```python
from build123d import *

# Parameters (mm, degrees)
SKETCH1_W           = 610
SKETCH1_H           = 200
SKETCH1_W_2         = 4
SKETCH1_H_2         = 20
SKETCH1_W_3         = 20
SKETCH1_H_3         = 4
BOSS_EXTRUDE1_DEPTH = 4
CUT_EXTRUDE1_DEPTH  = 10


with BuildPart() as part:
    # Sketch1 → Boss-Extrude1 (new body)
    with BuildSketch(Plane(origin=(0, 0, 0), x_dir=(1, 0, 0), z_dir=(0, 1, 0))):
        Rectangle(SKETCH1_W, SKETCH1_H)
        with Locations((-299, -85)):
            Rectangle(SKETCH1_W_2, SKETCH1_H_2, mode=Mode.SUBTRACT)
        with Locations((-299, 85)):
            Rectangle(SKETCH1_W_2, SKETCH1_H_2, mode=Mode.SUBTRACT)
        with Locations((-299, 0)):
            Rectangle(SKETCH1_W_2, SKETCH1_H_2, mode=Mode.SUBTRACT)
        with Locations((-275, 93)):
            Rectangle(SKETCH1_W_3, SKETCH1_H_3, mode=Mode.SUBTRACT)
        with Locations((-138, 93)):
            Rectangle(SKETCH1_W_3, SKETCH1_H_3, mode=Mode.SUBTRACT)
        with Locations((-1, 93)):
            Rectangle(SKETCH1_W_3, SKETCH1_H_3, mode=Mode.SUBTRACT)
        with Locations((-1, -93)):
            Rectangle(SKETCH1_W_3, SKETCH1_H_3, mode=Mode.SUBTRACT)
        with Locations((-138, -93)):
            Rectangle(SKETCH1_W_3, SKETCH1_H_3, mode=Mode.SUBTRACT)
        with Locations((-275, -93)):
            Rectangle(SKETCH1_W_3, SKETCH1_H_3, mode=Mode.SUBTRACT)
        with Locations((-49.859697176, -81)):
            Rectangle(SKETCH1_W_2, SKETCH1_H_2, mode=Mode.SUBTRACT)
        with Locations((-49.859697176, -32)):
            Rectangle(SKETCH1_W_2, SKETCH1_H_2, mode=Mode.SUBTRACT)
        with Locations((-64.859697176, -14)):
            Rectangle(SKETCH1_W_3, SKETCH1_H_3, mode=Mode.SUBTRACT)
        with Locations((-64.859697176, 14)):
            Rectangle(SKETCH1_W_3, SKETCH1_H_3, mode=Mode.SUBTRACT)
        with Locations((-49.859697176, 32)):
            Rectangle(SKETCH1_W_2, SKETCH1_H_2, mode=Mode.SUBTRACT)
        with Locations((0, -14)):
            Rectangle(SKETCH1_W_3, SKETCH1_H_3, mode=Mode.SUBTRACT)
        with Locations((0.140302824, 14)):
            Rectangle(SKETCH1_W_3, SKETCH1_H_3, mode=Mode.SUBTRACT)
        with Locations((136, 93)):
            Rectangle(SKETCH1_W_3, SKETCH1_H_3, mode=Mode.SUBTRACT)
        with Locations((273, 93)):
            Rectangle(SKETCH1_W_3, SKETCH1_H_3, mode=Mode.SUBTRACT)
        with Locations((49.859697176, -81)):
            Rectangle(SKETCH1_W_2, SKETCH1_H_2, mode=Mode.SUBTRACT)
        with Locations((49.859697176, -32)):
            Rectangle(SKETCH1_W_2, SKETCH1_H_2, mode=Mode.SUBTRACT)
        with Locations((64.859697176, -14)):
            Rectangle(SKETCH1_W_3, SKETCH1_H_3, mode=Mode.SUBTRACT)
        with Locations((64.859697176, 14)):
            Rectangle(SKETCH1_W_3, SKETCH1_H_3, mode=Mode.SUBTRACT)
        with Locations((49.859697176, 32)):
            Rectangle(SKETCH1_W_2, SKETCH1_H_2, mode=Mode.SUBTRACT)
        with Locations((273, -93)):
            Rectangle(SKETCH1_W_3, SKETCH1_H_3, mode=Mode.SUBTRACT)
        with Locations((136, -93)):
            Rectangle(SKETCH1_W_3, SKETCH1_H_3, mode=Mode.SUBTRACT)
        with Locations((49.859697176, 81)):
            Rectangle(SKETCH1_W_2, SKETCH1_H_2, mode=Mode.SUBTRACT)
        with Locations((-49.859697176, 81)):
            Rectangle(SKETCH1_W_2, SKETCH1_H_2, mode=Mode.SUBTRACT)
        with Locations((299, 85)):
            Rectangle(SKETCH1_W_2, SKETCH1_H_2, mode=Mode.SUBTRACT)
        with Locations((299, 0)):
            Rectangle(SKETCH1_W_2, SKETCH1_H_2, mode=Mode.SUBTRACT)
        with Locations((299, -85)):
            Rectangle(SKETCH1_W_2, SKETCH1_H_2, mode=Mode.SUBTRACT)
    extrude(amount=BOSS_EXTRUDE1_DEPTH)

    # Sketch2 → Cut-Extrude1 (cut)
    with BuildSketch(Plane(origin=(0, 4, 0), x_dir=(1, 0, 0), z_dir=(0, 1, 0))):
        Polygon((-47.859697176, 16), (47.859697176, 16), (47.859697176, 42), (74.859697176, 42), (107.419236847, 16), (107.419236847, -16), (74.859697176, -42), (47.859697176, -42), (47.859697176, -16), (-47.859697176, -16), (-47.859697176, -42), (-74.859697176, -42), (-107.419236847, -16), (-107.419236847, 16), (-74.859697176, 42), (-47.859697176, 42), align=None)
    extrude(amount=-CUT_EXTRUDE1_DEPTH, mode=Mode.SUBTRACT)


solid = part.part
```
Design review of the part built by this model. Coordinates are the model's own, in mm. A direction names the side the tool comes from. Round coordinates to 2 decimals unless told otherwise and drop trailing zeros. Order: outer loops, then holes, each group sorted by start corner. A loop starts at its lowest first (then second) coordinate and runs counter-clockwise, first axis right, second up. Notation, with made-up numbers: (0.25, 57.25) - (40.25, 57.25) arc R14 ccw to (40.25, 70.25) - close; hole circle Ø8 at (32.25, -37.5). An arc over 180 degrees is marked (long way). Return JSON: item names as keys, results as strings.
Q1. The part is to be moulded in two halves that separate along X. For faces 3 (the flat face through (-4, 4, -24)), 4 (the flat face through (91.367, 2.028, 28.818)), say which applies: pulls with the +X half, pulls with the -X half, needs draft (parallel to the pull), parting line crosses it, or undercut.
Computed values:
{"face 3": "needs draft", "face 4": "undercut"}
Q2. Consider section B-B on x = 40.5. Write out the cut boundary in (y, z).
Computed values:
{"outline": "(0, -100) - (4, -100) - (4, -16) - (0, -16) - close; (0, 16) - (4, 16) - (4, 100) - (0, 100) - close"}
Q3. Consider section D-D on y = 2.8. Give the number of separate pieces and of enclosed holes in the cut face, plus the area to 3 significant figures.
Computed values:
{"separate pieces": "1", "enclosed holes": "21", "area": "109,000 mm2"}
Q4. Consider section C-C on z = -32. Write out the cut boundary in (x, y).
Computed values:
{"outline": "(-305, 0) - (-87.38, 0) - (-87.38, 4) - (-305, 4) - close; (-47.86, 0) - (47.86, 0) - (47.86, 4) - (-47.86, 4) - close; (87.38, 0) - (305, 0) - (305, 4) - (87.38, 4) - close"}
Q5. For pin 1 Ø12 at (x, z) = (181, 24) entering from -Y, flat-tipped, find the tip position at first contact; note if it passes through.
Computed values:
{"pin 1": "stops at y = 0"}
Q6. Wall thickness on L1, parallel to X at y = 3, z = 74; L2, parallel to X at y = 2.8, z = -8; L3, parallel to Z at x = 134, y = 1.65: over which ranges is each line inside the solid? List them lowest first. Write a range as [from, to].
Computed values:
{"L1": "x = [-305, -51.86], [-47.86, 47.86], [51.86, 305]", "L2": "x = [-305, -301], [-297, -107.42], [107.42, 297], [301, 305]", "L3": "z = [-100, -95], [-91, 91], [95, 100]"}
Q7. Machinability: for faces 1 (the flat face through (-4, 0, -24)), 2 (the flat face through (90.912, 2.028, -29.182)), which of the approach directions +Z, -Z, +X, -X, +Y, -Y give a long, thin tool a straight path to every point of the face, cutting with its end or side? Answer none if there is none.
Computed values:
{"face 1": "+Z, -Z, +X, -X, -Y", "face 2": "+Y, -Y"}
Q8. Consider section A-A on z = 4. Write out the cut boundary in (x, y), plus the area to 3 significant figures.
Computed values:
{"outline": "(-305, 0) - (-301, 0) - (-301, 4) - (-305, 4) - close; (-297, 0) - (-107.42, 0) - (-107.42, 4) - (-297, 4) - close; (107.42, 0) - (297, 0) - (297, 4) - (107.42, 4) - close; (301, 0) - (305, 0) - (305, 4) - (301, 4) - close", "area": "1,550 mm2"}
